Design review of the part shown in the three views and the two pictorial views. Dimensions are in mm from the part's minimum x, y and z. A direction names the side the tool comes from. Coordinates: 2 decimals unless noted, no trailing zeros. Loops run counter-clockwise (first coordinate to the right, second up) from the corner with the lowest first, then second, coordinate; pieces in that order, holes last.
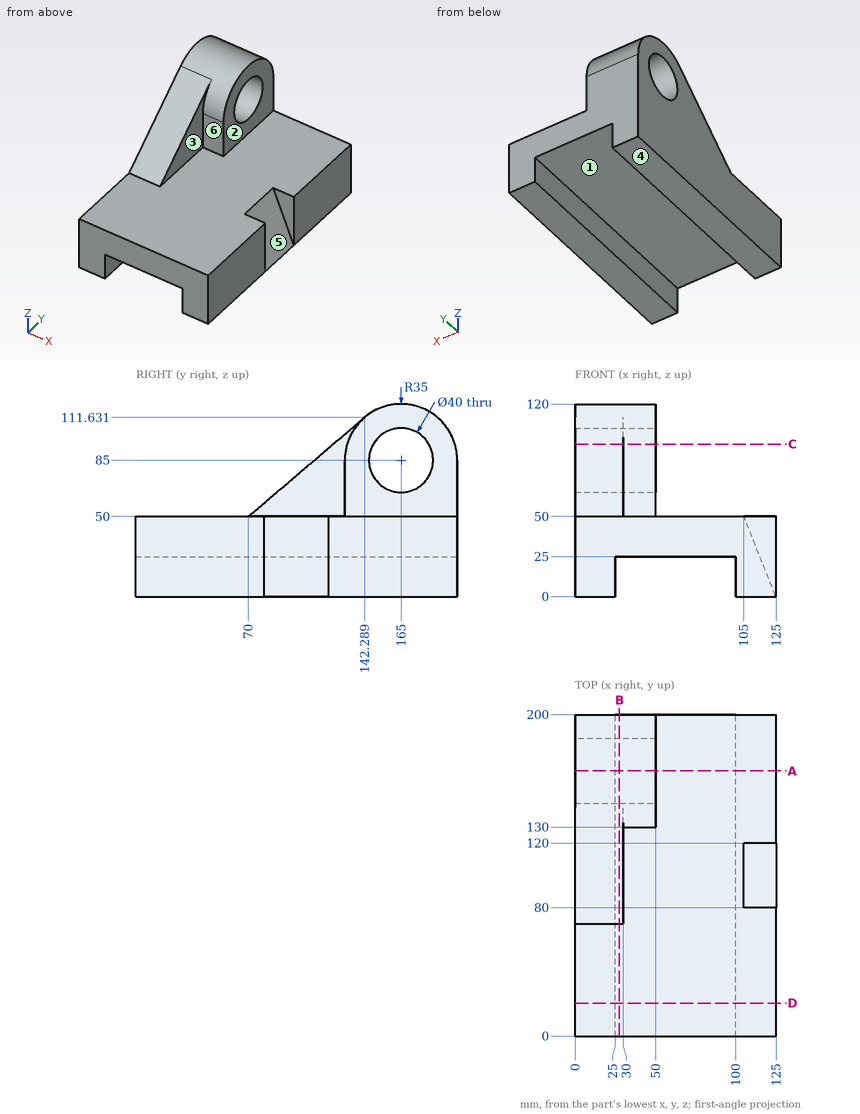
Q1. Consider section B-B (x = 27.5). State the section outline as (y, z) points.
Q2. For pin 1 Ø2 at (x, y) = (92.5, 131) entering from +Z; pin 2 Ø6 at (x, z) = (41, 68.5) entering from -Y; pin 3 Ø16 at (x, z) = (115, 33.5) entering from -Y; pin 4 Ø5 at (x, y) = (45.5, 23) entering from -Z, all flat-tipped, find the tip position at first contact; note any pin that passes through.
Q3. Consider section D-D (y = 20.5). State the section outline as (x, z) points.
Q4. Consider section A-A (y = 165). State the section outline as (x, z) points, then the cut area to 4 significant figures.
Q5. The part is to be moulded in two halves that separate along Y. For the marked faces 4, 5 and 6, say which applies: +Y half, -Y half, draft (parallel to the pull), parting line (faces both ways), or undercut.
Q6. Consider section C-C (z = 95). State the section outline as (x, y) points.
Q7. Machinability: for the marked faces 1, 2 and 3, which of the approach directions +Z, -Z, +X, -X, +Y, -Y give a long, thin tool a straight path to every point of the face, cutting with its end or side? Answer none if there is none.
Q8. Wall thickness on probe 1 along Z at (x, y) = (33, 165); probe 2 along Z at (x, y) = (21, 165); probe 3 along X at (y, z) = (139, 11.5): over which ranges is each line inside the solid? List them lowest first.
Model answer:
1. outline: (0, 25) - (200, 25) - (200, 85) arc R35 ccw to (142.29, 111.63) - (70, 50) - (0, 50) - close; hole circle Ø40 at (165, 85)
2. pin 1: stops at z = 50
2. pin 2: stops at y = 130
2. pin 3: stops at y = 0
2. pin 4: stops at z = 25
3. outline: (0, 0) - (25, 0) - (25, 25) - (100, 25) - (100, 0) - (125, 0) - (125, 50) - (0, 50) - close
4. outline: (0, 0) - (25, 0) - (25, 25) - (100, 25) - (100, 0) - (125, 0) - (125, 50) - (50, 50) - (50, 65) - (0, 65) - close; (0, 105) - (50, 105) - (50, 120) - (0, 120) - close
4. area: 5,875 mm2
5. face 4: draft
5. face 5: undercut
5. face 6: -Y half
6. outline: (0, 122.78) - (30, 122.78) - (30, 131.46) - (50, 131.46) - (50, 147.68) - (0, 147.68) - close; (0, 182.32) - (50, 182.32) - (50, 198.54) - (0, 198.54) - close
7. face 1: -Z, +Y, -Y
7. face 2: +Z, +X, +Y, -Y
7. face 3: +Z, +X, -Y
8. probe 1: z = 25 to 65, 105 to 120
8. probe 2: z = 0 to 65, 105 to 120
8. probe 3: x = 0 to 25, 100 to 125
